Autodesk Inventor part; units mm, degrees
ref_plane "YZ Plane" through (0, 0, 0) normal (1, 0, 0) x (0, 1, 0)
ref_plane "XZ Plane" through (0, 0, 0) normal (0, 1, 0) x (-1, 0, 0)
ref_plane "XY Plane" through (0, 0, 0) normal (0, 0, 1) x (1, 0, 0)
sketch "スケッチ1" plane through (0, 0, 0) normal (1, 0, 0) x (0, 1, 0)
  line L0 (0, 0) -> (15, 0)
  line L1 (15, 0) -> (15, -15)
  line L2 (15, -15) -> (0, -15)
  line L3 (0, -15) -> (0, 0)
  line L4 (14, -1) -> (1, -1)
  line L5 (1, -1) -> (1, -14)
  line L6 (1, -14) -> (14, -14)
  line L7 (14, -14) -> (14, -1)
  dimension "d0" = 15
  dimension "d1" = 15
  dimension "d2" = 1
extrude "押し出し1" add sketch "スケッチ1" along normal blind 450
sketch "スケッチ2" plane through (0, 0, 0) normal (0, 0, 1) x (1, 0, 0)
  line L0 (0, 15) -> (450, 15)
  line L1 (225, 15) -> (225, 0)
  line L2 (0, 15) -> (0, 0)
  point P0 (215, 7.5)
  point P1 (235, 7.5)
  dimension "d5" = 225
  dimension "d6" = 10
  dimension "d7" = 10
  dimension "d8" = 7.5
  dimension "d9" = 7.5
hole "穴1" at (215, 7.5, 0) at (235, 7.5, 0) direction (0, 0, -1) diameter 3 end through all
properties part number "hand-grab-v2-ASP-arm-support" material "アルミニウム 6061"
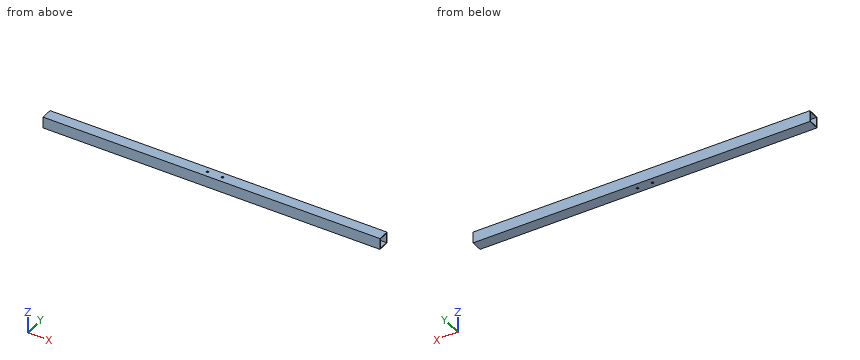
The model under review builds one solid part; all positions refer to its coordinate system, in mm. Round coordinates to 2 decimals unless told otherwise and drop trailing zeros. Loops run counter-clockwise (first coordinate to the right, second up) from the corner with the lowest first, then second, coordinate; pieces in that order, holes last. Notation, with made-up numbers: (-5.5, 75.5) -> (11.5, 75.5) arc R27 ccw to (11.5, 94.5) -> close; hole circle Ø9 at (89, 52.5). An arc over 180 degrees is marked (long way). Return JSON: item names as keys, results as strings.
(1) For line 1 (Z direction, x = 281, y = 4.5); line 2 (Y direction, x = 215, z = -14.55); line 3 (Y direction, x = 110.5, z = -6.75), list the stretches that pass through material, from the lowest coordinate up.
Solved:
{"line 1": "-15 to -14, -1 to 0", "line 2": "0 to 6, 9 to 15", "line 3": "0 to 1, 14 to 15"}
(2) Add section A-A on z = -8. Write out the cut boundary in (x, y).
Solved:
{"outline": "(0, 0) -> (450, 0) -> (450, 1) -> (0, 1) -> close; (0, 14) -> (450, 14) -> (450, 15) -> (0, 15) -> close"}
(3) For pin 1 (6.5 mm diameter, centred on x = 223, y = 10, fed in from +Z), flat-tipped, find the tip position at first contact; note if it passes through.
Solved:
{"pin 1": "z = 0"}
(4) Add section B-B on x = 315.5. Write out the cut boundary in (y, z).
Solved:
{"outline": "(0, -15) -> (15, -15) -> (15, 0) -> (0, 0) -> close; hole (1, -14) -> (14, -14) -> (14, -1) -> (1, -1) -> close"}
